from build123d import *

# Parameters (mm, degrees)
SKETCH_1_W          = 38.75
SKETCH_1_H          = 30
EXTRUDE_1_DEPTH     = 5
SKETCH_1_15_W       = 5
SKETCH_1_15_H       = 5
EXTRUDE_2_DEPTH     = 47
SKETCH_2_R          = 0.6
CUT_EXTRUDE_1_DEPTH = 66.177162411
SKETCH_3_R          = 1.5
SKETCH_3_R_2        = 0.75
CUT_EXTRUDE_2_DEPTH = 65.541169032
SKETCH_3_3_R        = 2.25
CUT_EXTRUDE_3_DEPTH = 3
SKETCH_4_W          = 5
SKETCH_4_H          = 42
EXTRUDE_3_DEPTH     = 2
EXTRUDE_START       = -5
SKETCH_4_3_W        = 5
SKETCH_4_3_H        = 42
EXTRUDE_4_DEPTH     = 2


with BuildPart() as part:
    # 草图1 → 凸台-拉伸1 (new body)
    with BuildSketch(Plane(origin=(0, 0, 0), x_dir=(1, 0, 0), z_dir=(0, 1, 0))):
        with Locations((-19.375, 15)):
            Rectangle(SKETCH_1_W, SKETCH_1_H)
    extrude(amount=EXTRUDE_1_DEPTH)

    # 草图1<15> → 凸台-拉伸2 (add)
    with BuildSketch(Plane(origin=(0, 0, 0), x_dir=(1, 0, 0), z_dir=(0, 1, 0))):
        with Locations((-2.5, 27.5)):
            Rectangle(SKETCH_1_15_W, SKETCH_1_15_H)
    extrude(amount=EXTRUDE_2_DEPTH)

    # 草图2 → 切除-拉伸1 (cut, through all)
    with BuildSketch(Plane.ZY.offset(5)):
        with Locations((-27.5, 42.5)):
            Circle(SKETCH_2_R)
    extrude(amount=-CUT_EXTRUDE_1_DEPTH, mode=Mode.SUBTRACT)

    # 草图3 → 切除-拉伸2 (cut, through all)
    with BuildSketch(Plane(origin=(0, 5, 0), x_dir=(1, 0, 0), z_dir=(0, 1, 0))):
        with Locations(Location((-9, 8, 0), (0, 0, 270))):
            Circle(SKETCH_3_R)
        with Locations(Location((-32.75, 8, 0), (0, 0, 270))):
            Circle(SKETCH_3_R)
        with Locations(Location((-19, 18, 0), (0, 0, 270))):
            Circle(SKETCH_3_R)
        with Locations(Location((-32.75, 18, 0), (0, 0, 270))):
            Circle(SKETCH_3_R_2)
        with Locations(Location((-9, 18, 0), (0, 0, 270))):
            Circle(SKETCH_3_R_2)
        with Locations(Location((-19, 8, 0), (0, 0, 270))):
            Circle(SKETCH_3_R_2)
    extrude(amount=-CUT_EXTRUDE_2_DEPTH, mode=Mode.SUBTRACT)

    # 草图3<3> → 切除-拉伸3 (cut)
    with BuildSketch(Plane(origin=(0, 5, 0), x_dir=(1, 0, 0), z_dir=(0, 1, 0))):
        with Locations(Location((-19, 18, 0), (0, 0, 270))):
            Circle(SKETCH_3_3_R)
        with Locations(Location((-32.75, 8, 0), (0, 0, 270))):
            Circle(SKETCH_3_3_R)
        with Locations(Location((-9, 8, 0), (0, 0, 270))):
            Circle(SKETCH_3_3_R)
    extrude(amount=-CUT_EXTRUDE_3_DEPTH, mode=Mode.SUBTRACT)

    # 草图4 → 凸台-拉伸3 (add)
    with BuildSketch(Plane.XY.offset(-25)):
        with Locations((-2.5, 26)):
            Rectangle(SKETCH_4_W, SKETCH_4_H)
    extrude(amount=EXTRUDE_3_DEPTH)

    # 草图4<3> → 凸台-拉伸4 (add)
    with BuildSketch(Plane.XY.offset(-25).offset(EXTRUDE_START)):
        with Locations((-2.5, 26)):
            Rectangle(SKETCH_4_3_W, SKETCH_4_3_H)
        Polygon((0, 0), (0, 5), (-5, 5), (-38.75, 5), (-38.75, 0), align=None)
    extrude(amount=-EXTRUDE_4_DEPTH)


solid = part.part
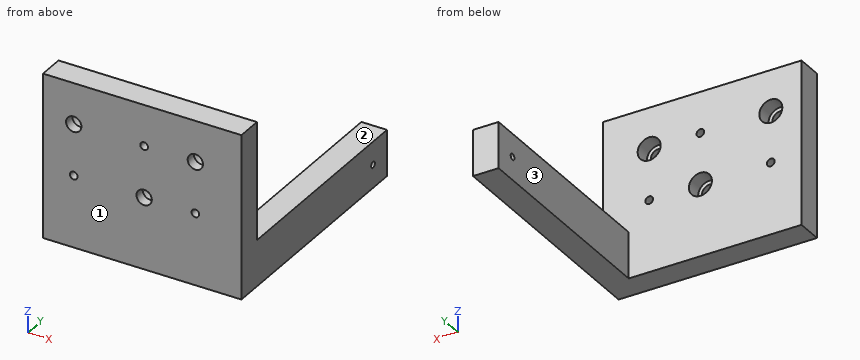
Geometry check sheet. Reference: the model listing, model coordinates, mm. Face numbers are marked on the shaded views. A direction names the side the tool comes from. Coordinates: 2 decimals unless noted, no trailing zeros. Order: outer loops, then holes, each group sorted by start corner. A loop starts at its lowest first (then second) coordinate and runs counter-clockwise, first axis right, second up. Notation, with made-up numbers: M 75,-36.5 L 94,-36.5 A29 ccw 94,-14.5 Z; hole C 58.25,59.5 d2. An arc over 180 degrees is marked long. Use CSV: the item, a comma, the result in double quotes.
Item 1: Thickness scan on line 1 along X through (y, z) = (1.25, -8); line 2 along X through (y, z) = (1, -18); line 3 along Z through (x, y) = (-3.05, 42.5). Record the ranges inside material, lowest first.
Returned:
line 1,"x = -38.75 to -34.25, -31.25 to -19.75, -18.25 to -10.5, -7.5 to 0"
line 2,"x = -38.75 to -33.5, -32 to -20.5, -17.5 to -9.75, -8.25 to 0"
line 3,"z = -32 to -28.1, -26.9 to -23"
Item 2: Tool access check on the marked faces 1, 2 and 3. Record the directions out of +Z, -Z, +X, -X, +Y, -Y that give a thin tool (end or side, any length) a straight path to the whole face; none if there is none.
Returned:
face 1,"+Z, -Z, +X, -X, -Y"
face 2,"+Z, +X, -X, +Y"
face 3,"+Z, -Z, -X, +Y"
Item 3: Gauge pin test, flat ends, axial feed: pin 1 Ø4 at (x, z) = (-9, -8) entering from +Y; pin 2 Ø8 at (y, z) = (41.5, -25) entering from -X; pin 3 Ø3.5 at (x, z) = (-32, -7.5) entering from +Y. Record the tip position at first contact, or that the pin passes through.
Returned:
pin 1,"stops at y = 2"
pin 2,"stops at x = -5"
pin 3,"stops at y = 5"
Item 4: Cross-section at B-B on x = -32.75. Record the cut outline in (y, z).
Returned:
outline,"M 0,-32 L 5,-32 L 5,-18.75 L 0,-18.75 Z; M 0,-17.25 L 5,-17.25 L 5,-10.25 L 2,-10.25 L 2,-9.5 L 0,-9.5 Z; M 0,-6.5 L 2,-6.5 L 2,-5.75 L 5,-5.75 L 5,0 L 0,0 Z"
Item 5: Cross-section at A-A on z = -27.5. Record the cut outline in (x, y).
Returned:
outline,"M -38.75,0 L 0,0 L 0,41.9 L -5,41.9 L -5,5 L -38.75,5 Z; M -5,43.1 L 0,43.1 L 0,47 L -5,47 Z"
Item 6: Cross-section at D-D on z = -18. Record the cut outline in (x, y), then the cut area to 3 significant figures.
Returned:
outline,"M -38.75,0 L -33.5,0 L -33.5,5 L -38.75,5 Z; M -32,0 L -20.5,0 L -20.5,2 L -21.25,2 L -21.25,5 L -32,5 Z; M -17.5,0 L -9.75,0 L -9.75,5 L -16.75,5 L -16.75,2 L -17.5,2 Z; M -8.25,0 L 0,0 L 0,5 L -8.25,5 Z"
area,"159 mm2"
Item 7: Cross-section at C-C on y = 42.5. Record the cut outline in (x, z), then the cut area to 3 significant figures.
Returned:
outline,"M -5,-32 L 0,-32 L 0,-28.1 L -5,-28.1 Z; M -5,-26.9 L 0,-26.9 L 0,-23 L -5,-23 Z"
area,"39.0 mm2"
